```python
from build123d import *

# Parameters (mm, degrees)
SKETCH1_R            = 8
BOSS_EXTRUDE1_DEPTH  = 10
M6_CLEARANCE_HOLE1_D = 6.6


with BuildPart() as part:
    # Sketch1 → Boss-Extrude1 (new body)
    with BuildSketch(Plane.XY):
        with BuildLine():
            Line((-14, 19.5), (14, 19.5))
            ThreePointArc((14, 19.5), (24.005207768, 0), (14, -19.5))
            Line((14, -19.5), (-14, -19.5))
            ThreePointArc((-14, -19.5), (-24.005207768, 0), (-14, 19.5))
        make_face()
        Circle(SKETCH1_R, mode=Mode.SUBTRACT)
    extrude(amount=BOSS_EXTRUDE1_DEPTH)

    # M6 Clearance Hole1 (through all)
    with Locations(Plane.XY.offset(10)):
        with Locations((-13.435028843, 13.435028843), (13.435028843, 13.435028843), (19, 0), (13.435028843, -13.435028843), (-13.435028843, -13.435028843), (-19, 0)):
            Hole(M6_CLEARANCE_HOLE1_D / 2)


solid = part.part
```
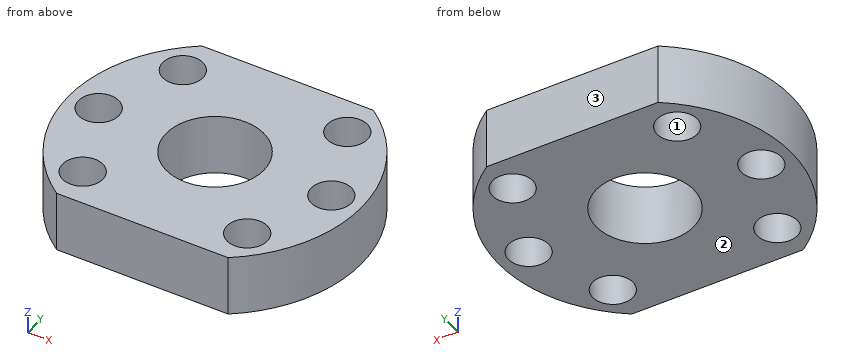
The model under review builds one solid part; all positions refer to its coordinate system, in mm. Face numbers are marked on the shaded views. Round coordinates to 2 decimals unless told otherwise and drop trailing zeros. Order: outer loops, then holes, each group sorted by start corner. A loop starts at its lowest first (then second) coordinate and runs counter-clockwise, first axis right, second up.
Item 1: Add section B-B, the plane y = 0. State the section outline as (x, z) points, and give its area (3 significant figures).
Working result:
outline: (-24.01, 0) - (-22.3, 0) - (-22.3, 10) - (-24.01, 10) - close; (-15.7, 0) - (-8, 0) - (-8, 10) - (-15.7, 10) - close; (8, 0) - (15.7, 0) - (15.7, 10) - (8, 10) - close; (22.3, 0) - (24.01, 0) - (24.01, 10) - (22.3, 10) - close
area: 188 mm2
Item 2: For pin 1 (5 mm diameter, centred on x = -18.5, z = 5, fed in from -Y); pin 2 (1 mm diameter, centred on y = 10, z = 4.5, fed in from -X); pin 3 (1.5 mm diameter, centred on y = -5.5, z = 4, fed in from +X), all flat-tipped, find the tip position at first contact; note any pin that passes through.
Working result:
pin 1: stops at y = -17.9
pin 2: stops at x = -22.05
pin 3: stops at x = 23.53
Item 3: To check wall thickness, follow probe 1 along Y at (x, z) = (12.5, 3.25); probe 2 along Y at (x, z) = (-11, 7.5); probe 3 along X at (y, z) = (-1, 7.5). State the ranges of each line that lie inside material, in increasing order.
Working result:
probe 1: y = -19.5 to -16.6, -10.27 to 10.27, 16.6 to 19.5
probe 2: y = -19.5 to -15.66, -11.21 to 11.21, 15.66 to 19.5
probe 3: x = -23.98 to -22.14, -15.86 to -7.94, 7.94 to 15.86, 22.14 to 23.98
Item 4: Add section D-D, the plane z = 4.25. State the section outline as (x, y) points.
Working result:
outline: (-14, -19.5) - (14, -19.5) arc R24.01 ccw to (14, 19.5) - (-14, 19.5) arc R24.01 ccw to start; hole circle Ø6.6 at (-19, 0); hole circle Ø6.6 at (-13.44, -13.44); hole circle Ø6.6 at (-13.44, 13.44); hole circle Ø16 at (0, 0); hole circle Ø6.6 at (13.44, -13.44); hole circle Ø6.6 at (13.44, 13.44); hole circle Ø6.6 at (19, 0)
Item 5: Add section A-A, the plane x = 0. State the section outline as (y, z) points.
Working result:
outline: (-19.5, 0) - (-8, 0) - (-8, 10) - (-19.5, 10) - close; (8, 0) - (19.5, 0) - (19.5, 10) - (8, 10) - close
Item 6: Add section C-C, the plane y = -6. State the section outline as (x, z) points, and give its area (3 significant figures).
Working result:
outline: (-23.24, 0) - (-5.29, 0) - (-5.29, 10) - (-23.24, 10) - close; (5.29, 0) - (23.24, 0) - (23.24, 10) - (5.29, 10) - close
area: 359 mm2
Item 7: Draft analysis for pull direction Y (two halves, no side actions). For the marked faces 1, 2 and 3, state which applies: released by +Y, released by -Y, zero draft, split by the parting line, or undercut.
Working result:
face 1: undercut
face 2: zero draft
face 3: released by +Y
